Part model, mm, in its own coordinate system. Face numbers are marked on the shaded views. A direction names the side the tool comes from. Give positions to 0.01 mm unless a question says otherwise; leave off trailing zeros. Write each loop counter-clockwise with the first axis right and the second up, starting at its lowest first coordinate (ties: lowest second). Pieces come first, ordered by that corner, then holes. Notation, with made-up numbers: M 36.25,-18 L 53.25,-18 A16 cw 53.25,-9 Z; hole C 48,79.25 d4. An arc over 180 degrees is marked long. Write item = value, one per line. Start each with the question number.
from build123d import *

# Parameters (mm, degrees)
F1_DEPTH     = 5
F3_DEPTH     = 20
F5_DEPTH     = 40
F6_W         = 20
F6_H         = 20
F7_DEPTH     = 20
F8_R         = 1.5
F12_D        = 4.2
F12_ON_F11_D = 4.2
F12_ON_F10_D = 4.2


with BuildPart() as f1:
    # F0 (on Top) → F1 (new body)
    with BuildSketch(Plane.XY):
        with BuildLine():
            Line((-65, 0), (0, 0))
            Line((0, 0), (0, 65))
            Line((0, 65), (-25, 65))
            ThreePointArc((-25, 65), (-38.7994204149, 38.7994204149), (-65, 25))
            Line((-65, 25), (-65, 0))
        make_face()
    extrude(amount=F1_DEPTH)

    # F2 (on face) → F3 (join)
    with BuildSketch(Plane.XY.offset(5)):
        Polygon((-25, 25), (-65, 25), (-65, 20), (-25, 20), (-25, 0), (-20, 0), (-20, 20), (0, 20), (0, 25), (-20, 25), (-20, 65), (-25, 65), align=None)
    extrude(amount=F3_DEPTH)

    # F4 (on face) → F5 (join)
    with BuildSketch(Plane.XY.offset(25)):
        Polygon((0, 25), (-25, 25), (-25, 0), (-20, 0), (-20, 20), (0, 20), align=None)
    extrude(amount=F5_DEPTH)

    # F6 (on face) → F7 (join)
    with BuildSketch(Plane.XY.offset(5)):
        with Locations((-10, 10)):
            Rectangle(F6_W, F6_H)
    extrude(amount=F7_DEPTH)

    # F8
    f8_edges = [f1.edges().sort_by_distance(p)[0] for p in [
        (0, 0, 12.5),
    ]]
    fillet(f8_edges, radius=F8_R)

    # F12 (through all)
    with Locations(Plane.XZ.offset(-20)):
        with Locations((-55, 15), (-35, 15), (-10, 35), (-10, 55)):
            Hole(F12_D / 2)

    # F12 on F11 (through all)
    with Locations(Plane.XY.offset(5)):
        with Locations((-35, 10), (-55, 10), (-10, 55), (-10, 35)):
            Hole(F12_ON_F11_D / 2)

    # F12 on F10 (through all)
    with Locations(Plane.YZ.offset(-20)):
        with Locations((10, 35), (10, 55), (35, 15), (55, 15)):
            Hole(F12_ON_F10_D / 2)


solid = f1.part
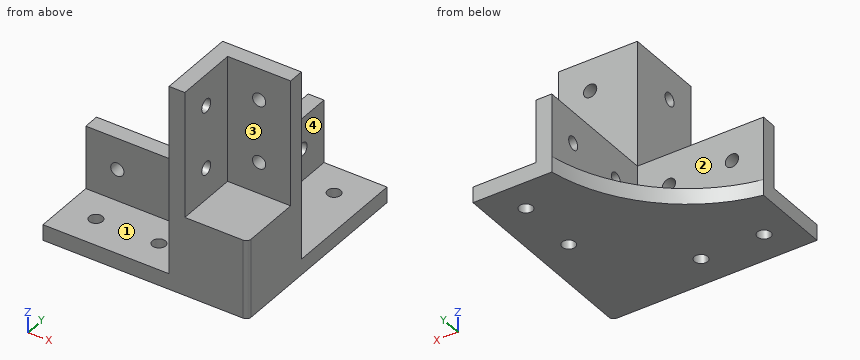
Q1. Drop flat-ended pins along their axis: P1, Ø4, axis at x = -7.5, z = 55, coming from the -Y side; P2, Ø2, axis at x = -30, y = 14.5, coming from the +Z side; P3, Ø8, axis at y = 50, z = 17.5, coming from the +X side; P4, Ø4, axis at x = -55, z = 15, coming from the -Y side. Give the stop position or say it passes through.
Q2. Slice it at C-C (z = 35). Give the cut face in (x, y).
Q3. Tool access for the marked faces 1, 2, 3 and 4: list every direction of +Z, -Z, +X, -X, +Y, -Y with a clear straight run to the whole face (end or side of a thin tool).
Q4. Slice it at A-A (y = 10). Give the cut face in (x, z).
Q5. Probe line 1 along Z through (x, y) = (-21.55, 35); line 2 along X through (y, z) = (16, 52); line 3 along Z through (x, y) = (-21, 45). List the from-to ranges inside material, lowest first.
Q6. Slice it at B-B (z = 15). Give the cut face in (x, y).
Q7. Slice it at D-D (x = -10). Give the cut face in (y, z), and give its area (3 significant figures).
Working result:
q1.P1 = 20
q1.P2 = 5
q1.P3 = -20
q1.P4 = through
q2.outline = M -25,0 L -20,0 L -20,7.9 L -25,7.9 Z; M -25,12.1 L -20,12.1 L -20,20 L -12.1,20 L -12.1,25 L -25,25 Z; M -7.9,20 L 0,20 L 0,25 L -7.9,25 Z
q3.face_1 = +Z, -X, -Y
q3.face_2 = +Z, -X, +Y
q3.face_3 = +Z, +X, -Y
q3.face_4 = +Z, +X, +Y
q4.outline = M -65,0 L -57.1,0 L -57.1,5 L -65,5 Z; M -52.9,0 L -37.1,0 L -37.1,5 L -52.9,5 Z; M -32.9,0 L 0,0 L 0,25 L -20,25 L -20,32.9 L -25,32.9 L -25,5 L -32.9,5 Z; M -25,37.1 L -20,37.1 L -20,52.9 L -25,52.9 Z; M -25,57.1 L -20,57.1 L -20,65 L -25,65 Z
q5.line_1 = 0 to 12.9, 17.1 to 25
q5.line_2 = -25 to -20
q5.line_3 = 0 to 25
q6.outline = M -65,20 L -57.1,20 L -57.1,25 L -65,25 Z; M -52.9,20 L -37.1,20 L -37.1,25 L -52.9,25 Z; M -32.9,20 L -25,20 L -25,0 L -1.5,0 A1.5 ccw 0,1.5 L 0,25 L -20,25 L -20,32.9 L -25,32.9 L -25,25 L -32.9,25 Z; M -25,37.1 L -20,37.1 L -20,52.9 L -25,52.9 Z; M -25,57.1 L -20,57.1 L -20,65 L -25,65 Z
q7.outline = M 0,0 L 32.9,0 L 32.9,5 L 25,5 L 25,32.9 L 20,32.9 L 20,25 L 0,25 Z; M 20,37.1 L 25,37.1 L 25,52.9 L 20,52.9 Z; M 20,57.1 L 25,57.1 L 25,65 L 20,65 Z; M 37.1,0 L 52.9,0 L 52.9,5 L 37.1,5 Z; M 57.1,0 L 65,0 L 65,5 L 57.1,5 Z
q7.area = 941 mm2
